Autodesk Inventor part; units mm, degrees
ref_plane "YZ Plane" through (0, 0, 0) normal (1, 0, 0) x (0, 1, 0)
ref_plane "XZ Plane" through (0, 0, 0) normal (0, 1, 0) x (-1, 0, 0)
ref_plane "XY Plane" through (0, 0, 0) normal (0, 0, 1) x (1, 0, 0)
sketch "Boceto1" plane through (0, 0, 0) normal (0, 0, 1) x (1, 0, 0)
  circle A0 centre (0, 0) radius 30.35
  circle A1 centre (0, 0) radius 35
  circle A2 centre (0, 0) radius 27.35
  circle A3 centre (0, 0) radius 37
  dimension "d0" = 60.7
  dimension "d1" = 70
  dimension "d2" = 3
  dimension "d3" = 2
extrude "Extrusión1" add sketch "Boceto1" along normal blind 10
sketch "Boceto2" plane through (0, 0, 0) normal (0, 0, -1) x (-1, 0, 0)
  circle A0 centre (0, 0) radius 30.35
  circle A1 centre (0, 0) radius 35
  circle A2 centre (0, 0) radius 37
extrude "Extrusión2" add sketch "Boceto2" along normal blind 4 contours A0 | A1 | A2
sketch "Boceto3" plane through (0, 0, -4) normal (0, 0, -1) x (-1, 0, 0)
  circle A0 centre (0, 0) radius 2
  dimension "d8" = 4
extrude "Extrusión3" cut sketch "Boceto3" against normal blind 4
properties part number "base_estable_soporte_3DPrint"
Read the model definition and answer for the solid it produces. Units are mm, in the model's axes. A direction names the side the tool comes from. Give positions to 0.01 mm unless a question says otherwise; leave off trailing zeros. Write each loop counter-clockwise with the first axis right and the second up, starting at its lowest first coordinate (ties: lowest second). Pieces come first, ordered by that corner, then holes. Notation, with made-up numbers: (82.5, 83.5) -> (134.5, 83.5) arc R8 ccw to (134.5, 91.5) -> close; hole circle Ø2 at (-25.75, 58.25). An arc over 180 degrees is marked (long way). Answer as a JSON object with one key per item and string values. Group by question number.
1) Find section D-D (z = -1.25). Write down the section's boundary in (x, y).
2) A tool of negligible diameter and unlimited length cuts with its end or side. For faces 4 (the flat face through (0, -6, 0)), 5 (the flat face through (-27.12, 4.64, 10)), from which of +Z, -Z, +X, -X, +Y, -Y can it reach the whole face along a straight path? Write none if from no direction.
3) Each of these flat-tipped pins is pushed along its axis until it touches: P1, Ø2, axis at x = -13.5, y = 27.5, coming from the +Z side; P2, Ø5, axis at x = 23, z = 1, coming from the -Y side; P3, Ø6, axis at x = 9.5, z = 4, coming from the -Y side; P4, Ø5, axis at x = 9.5, z = 2.5, coming from the -Y side. Where does it stop, or does it pass through?
4) Find section B-B (y = 1). Write down the section's boundary in (x, z), and give its area (3 significant figures).
5) The mould has two halves that part along Y. Classify faces 1 (the flat face through (-8, 1, -4)), 2 (the flat face through (11, 29, 0)), 3 (the cylindrical face through (0, -2, -2)): +Y half, -Y half, draft (parallel to the pull), parting line (faces both ways), or undercut.
6) Find section C-C (x = 0). Write down the section's boundary in (y, z).
7) Find section A-A (z = 5.25). Write down the section's boundary in (x, y), and give its area (3 significant figures).
8) Consider L1, parallel to Y at x = 0, z = 7.25; L2, parallel to X at y = -14.5, z = 3.25; L3, parallel to X at y = -2.5, z = 2.25. Determine where each line is inside the solid, lowest interval first. Write a range as from..to.
Values follow:
{
 "1": {"outline": "circle Ø74 at (0, 0); hole circle Ø4 at (0, 0)"},
 "2": {"face 4": "+Z", "face 5": "+Z, +X, -X, +Y, -Y"},
 "3": {"P1": "stops at z = 10", "P2": "stops at y = -30.8", "P3": "stops at y = -36.42", "P4": "stops at y = -36.33"},
 "4": {"outline": "(-36.99, -4) -> (-1.73, -4) -> (-1.73, 0) -> (-27.33, 0) -> (-27.33, 10) -> (-30.33, 10) -> (-30.33, 0) -> (-34.99, 0) -> (-34.99, 10) -> (-36.99, 10) -> close; (1.73, -4) -> (36.99, -4) -> (36.99, 10) -> (34.99, 10) -> (34.99, 0) -> (30.33, 0) -> (30.33, 10) -> (27.33, 10) -> (27.33, 0) -> (1.73, 0) -> close", "area": "382 mm2"},
 "5": {"face 1": "draft", "face 2": "undercut", "face 3": "undercut"},
 "6": {"outline": "(-37, -4) -> (-2, -4) -> (-2, 0) -> (-27.35, 0) -> (-27.35, 10) -> (-30.35, 10) -> (-30.35, 0) -> (-35, 0) -> (-35, 10) -> (-37, 10) -> close; (2, -4) -> (37, -4) -> (37, 10) -> (35, 10) -> (35, 0) -> (30.35, 0) -> (30.35, 10) -> (27.35, 10) -> (27.35, 0) -> (2, 0) -> close"},
 "7": {"outline": "circle Ø74 at (0, 0); circle Ø60.7 at (0, 0); hole circle Ø70 at (0, 0); hole circle Ø54.7 at (0, 0)", "area": "996 mm2"},
 "8": {"L1": "y = -37..-35, -30.35..-27.35, 27.35..30.35, 35..37", "L2": "x = -34.04..-31.86, -26.66..-23.19, 23.19..26.66, 31.86..34.04", "L3": "x = -36.92..-34.91, -30.25..-27.24, 27.24..30.25, 34.91..36.92"}
}
